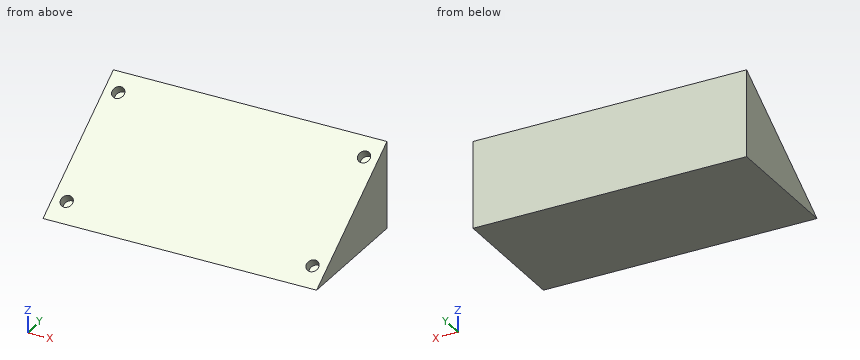
from build123d import *

# Parameters (mm, degrees)
F1_DEPTH = 31.5
F2_R     = 0.7
F3_DEPTH = 1.1


with BuildPart() as f1:
    # F0 (on Right) → F1 (new body)
    with BuildSketch(Plane.YZ):
        Polygon((14.846212, 0), (14.846212, 10), (0, 0), align=None)
    extrude(amount=F1_DEPTH)

    # F2 (on face) → F3 (cut)
    with BuildSketch(Plane(origin=(0, 0, 0), x_dir=(1, 0, 0), z_dir=(0, -0.558659, 0.829397))):
        with Locations((1.6, 15.6)):
            Circle(F2_R)
        with Locations((29.9, 15.6)):
            Circle(F2_R)
        with Locations((29.9, 2.5)):
            Circle(F2_R)
        with Locations((1.6, 2.5)):
            Circle(F2_R)
    extrude(amount=-F3_DEPTH, mode=Mode.SUBTRACT)


solid = f1.part
Verification items for the finished model (mm, model axes). Give positions to 0.01 mm unless a question says otherwise; leave off trailing zeros. Write each loop counter-clockwise with the first axis right and the second up, starting at its lowest first coordinate (ties: lowest second). Pieces come first, ordered by that corner, then holes.
(1) Cross-section at A-A (x = 12.5). Enter the section's corners in (y, z).
(2) Cross-section at C-C (z = 4.5). Enter the section's corners in (x, y).
(3) Cross-section at B-B (y = 12). Enter the section's corners in (x, z).
(4) Material ranges on line 1 (Z direction, x = 29, y = 11); line 2 (Y direction, x = 4, z = 0.5); line 3 (Z direction, x = 5, y = 2.5), recorded low to high.
(5) Gauge pin test, flat ends, axial feed: pin 1 (5 mm diameter, centred on x = 26.5, y = 6, fed in from +Z); pin 2 (3 mm diameter, centred on x = 6.5, z = 2.5, fed in from -Y). Record the tip position at first contact, or that the pin passes through.
Worked out:
1. outline: (0, 0) - (14.85, 0) - (14.85, 10) - close
2. outline: (0, 6.68) - (31.5, 6.68) - (31.5, 14.85) - (0, 14.85) - close
3. outline: (0, 0) - (31.5, 0) - (31.5, 8.08) - (0, 8.08) - close
4. line 1: z = 0 to 7.41
4. line 2: y = 0.74 to 14.85
4. line 3: z = 0 to 1.68
5. pin 1: stops at z = 5.73
5. pin 2: stops at y = 1.48
